```python
from build123d import *

# Parameters (mm, degrees)
SKETCH_1_W          = 41.58
SKETCH_1_H          = 4.8
SKETCH_1_R          = 1.15
EXTRUDE_1_DEPTH     = 3
SKETCH_2_R          = 2.05
CUT_EXTRUDE_1_DEPTH = 1.2


with BuildPart() as part:
    # 草图1 → 凸台-拉伸1 (new body)
    with BuildSketch(Plane(origin=(0, 0, 0), x_dir=(0, 0, -1), z_dir=(1, 0, 0))):
        with Locations((20.79, 2.4)):
            Rectangle(SKETCH_1_W, SKETCH_1_H)
        with Locations((14.79, 2.4)):
            Circle(SKETCH_1_R, mode=Mode.SUBTRACT)
        with Locations((5.79, 2.4)):
            Circle(SKETCH_1_R, mode=Mode.SUBTRACT)
        with Locations(Location((26.79, 2.4, 0), (0, 0, 180))):
            Circle(SKETCH_1_R, mode=Mode.SUBTRACT)
        with Locations(Location((35.79, 2.4, 0), (0, 0, 180))):
            Circle(SKETCH_1_R, mode=Mode.SUBTRACT)
    extrude(amount=EXTRUDE_1_DEPTH)

    # 草图2 → 切除-拉伸1 (cut)
    with BuildSketch(Plane(origin=(3, 0, 0), x_dir=(0, 0, -1), z_dir=(1, 0, 0))):
        with Locations((5.79, 2.4)):
            Circle(SKETCH_2_R)
        with Locations((14.79, 2.4)):
            Circle(SKETCH_2_R)
        with Locations((26.79, 2.4)):
            Circle(SKETCH_2_R)
        with Locations((35.79, 2.4)):
            Circle(SKETCH_2_R)
    extrude(amount=-CUT_EXTRUDE_1_DEPTH, mode=Mode.SUBTRACT)


solid = part.part
```
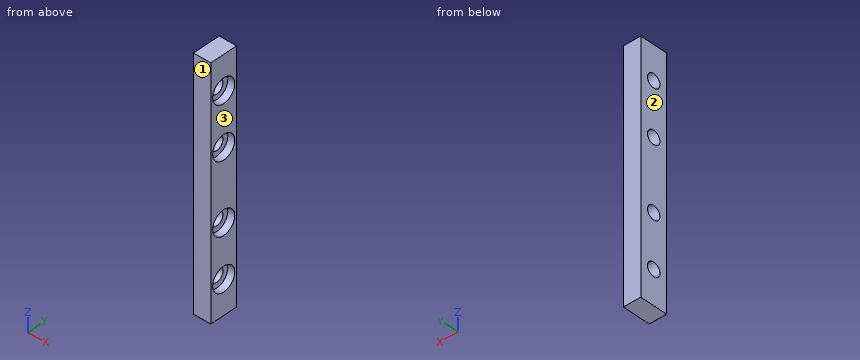
Design review of the part built by this model. Coordinates are the model's own, in mm. Face numbers are marked on the shaded views. Round coordinates to 2 decimals unless told otherwise and drop trailing zeros. Order: outer loops, then holes, each group sorted by start corner. A loop starts at its lowest first (then second) coordinate and runs counter-clockwise, first axis right, second up. Notation, with made-up numbers: M 35.25,42 L 58.25,42 A15 cw 58.25,52 Z; hole C 30,1.5 d5. An arc over 180 degrees is marked long. Put each result on its own line as item: value.
Q1. Insertion check: pin 1 Ø2.5 at (y, z) = (2.4, -35.79) entering from +X. The pin has a flat end and moves straight along its axis. Give the tip position at first contact, or say it passes through.
Reported:
pin 1: x = 1.8
Q2. Draft analysis for pull direction X (two halves, no side actions). For the marked faces 1, 2 and 3, state which applies: released by +X, released by -X, zero draft, split by the parting line, or undercut.
Reported:
face 1: zero draft
face 2: released by -X
face 3: released by +X
Q3. Consider section C-C (y = 2.4). State how many separate pieces and enclosed holes the cut face has, and give its area (3 significant figures).
Reported:
separate pieces: 5
enclosed holes: 0
area: 88.5 mm²
Q4. To check wall thickness, follow line 1 (Z direction, x = 0.6, y = 2.5); line 2 (Y direction, x = 2.5, z = -14.79); line 3 (Z direction, x = 1.9, y = 3.35). State the ranges of each line that lie inside material, in increasing order.
Reported:
line 1: -41.58 to -36.94, -34.64 to -27.94, -25.64 to -15.94, -13.64 to -6.94, -4.64 to 0
line 2: 0 to 0.35, 4.45 to 4.8
line 3: -41.58 to -37.61, -33.97 to -28.61, -24.97 to -16.61, -12.97 to -7.61, -3.97 to 0
Q5. Consider section D-D (z = -28.5). State the section outline as (x, y) points, and give its area (3 significant figures).
Reported:
outline: M 0,0 L 3,0 L 3,1.27 L 1.8,1.27 L 1.8,3.53 L 3,3.53 L 3,4.8 L 0,4.8 Z
area: 11.7 mm²
Q6. Consider section B-B (x = 2.4). State the section outline as (y, z) points.
Reported:
outline: M 0,-41.58 L 4.8,-41.58 L 4.8,0 L 0,0 Z; hole C 2.4,-35.79 d4.1; hole C 2.4,-26.79 d4.1; hole C 2.4,-14.79 d4.1; hole C 2.4,-5.79 d4.1
Q7. Consider section A-A (z = -35.79). State the section outline as (x, y) points.
Reported:
outline: M 0,0 L 3,0 L 3,0.35 L 1.8,0.35 L 1.8,1.25 L 0,1.25 Z; M 0,3.55 L 1.8,3.55 L 1.8,4.45 L 3,4.45 L 3,4.8 L 0,4.8 Z
